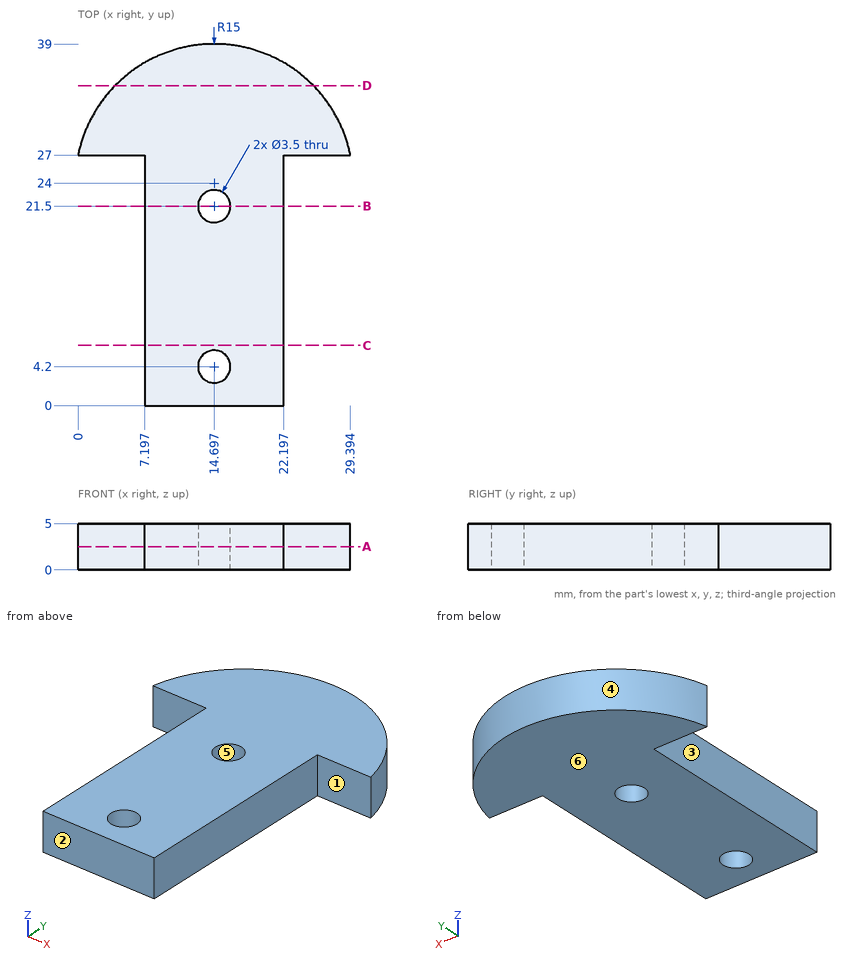
Could you check a few things on this drawing? It's one solid part, dimensions in mm from its lowest x, y, z. A direction names the side the tool comes from. Coordinates: 2 decimals unless noted, no trailing zeros. Write each loop counter-clockwise with the first axis right and the second up, starting at its lowest first coordinate (ties: lowest second). Pieces come first, ordered by that corner, then holes. Notation, with made-up numbers: M 14,28.25 L 71,28.25 A16 ccw 71,44.25 Z; hole C 41,-27 d4. An arc over 180 degrees is marked long. Answer as CSV lines item,"result". Start each with the question number.
Q1. Suppose I cut it at C-C, the plane y = 6.5. List the corners of the cut face in (x, z) for me, then the cut area to 3 significant figures.
Q2. Will these pins go through, and if not, where does the flat tip stop? pin 1 Ø2.5 at (y, z) = (10.5, 3) entering from +X; pin 2 Ø3 at (x, y) = (14.7, 4.2) entering from -Z.
Q3. Suppose I cut it at D-D, the plane y = 34.5. List the corners of the cut face in (x, z) for me (3 decimals).
Q4. I need wall thicknesses on probe 1 along Y at (x, z) = (15.5, 3.65) (1 decimal); probe 2 along X at (y, z) = (2, 3.1); probe 3 along X at (y, z) = (3.5, 0.3). Which ranges of each line are inside material? Lowest first, please. Write a range as [from, to].
Q5. Suppose I cut it at A-A, the plane z = 2.5. List the corners of the cut face in (x, y) for me, then the cut area to 3 significant figures.
Q6. If we mould it in two halves opening along X, with no side actions, what happens to the marked faces 4, 5 and 6? For each: pulls with the +X half, pulls with the -X half, needs draft (parallel to the pull), parting line crosses it, or undercut.
Q7. For the marked faces 1, 2 and 3, which set-ups out of +Z, -Z, +X, -X, +Y, -Y let a thin tool reach every point of the face, with its end or its side?
Q8. Suppose I cut it at B-B, the plane y = 21.5. List the corners of the cut face in (x, z) for me.
Entries:
1,outline,"M 7.2,0 L 22.2,0 L 22.2,5 L 7.2,5 Z"
1,area,"75.0 mm²"
2,pin 1,"stops at x = 22.2"
2,pin 2,"passes through"
3,outline,"M 3.985,0 L 25.409,0 L 25.409,5 L 3.985,5 Z"
4,probe 1,"y = [0, 2.6], [5.8, 19.9], [23.1, 39]"
4,probe 2,"x = [7.2, 22.2]"
4,probe 3,"x = [7.2, 13.09], [16.3, 22.2]"
5,outline,"M 0,27 L 7.2,27 L 7.2,0 L 22.2,0 L 22.2,27 L 29.39,27 A15 ccw Z; hole C 14.7,4.2 d3.5; hole C 14.7,21.5 d3.5"
5,area,"650 mm²"
6,face 4,"parting line crosses it"
6,face 5,"undercut"
6,face 6,"needs draft"
7,face 1,"+Z, -Z, +X, -Y"
7,face 2,"+Z, -Z, +X, -X, -Y"
7,face 3,"+Z, -Z, -X, -Y"
8,outline,"M 7.2,0 L 12.95,0 L 12.95,5 L 7.2,5 Z; M 16.45,0 L 22.2,0 L 22.2,5 L 16.45,5 Z"
